Could you check a few things on this model? Use its own coordinates, in mm. Face numbers are marked on the shaded views. Round coordinates to 2 decimals unless told otherwise and drop trailing zeros. Loops run counter-clockwise (first coordinate to the right, second up) from the corner with the lowest first, then second, coordinate; pieces in that order, holes last. Notation, with made-up numbers: (59, 57) - (111, 57) arc R17 ccw to (111, 72) - close; hole circle Ø4 at (22.5, -25.5). An arc over 180 degrees is marked (long way). Answer as CSV lines item,"result". Start each with the question number.
1) Suppose I cut it at C-C, the plane y = -4. Write out the boundary of the cut face in (x, z), then the cut area to 3 significant figures.
2) Please list where these lines run through material, in increasing order: line 1 along X through (y, z) = (-3.65, 0); line 2 along Z through (x, y) = (59.43, -2.5); line 3 along X through (y, z) = (0.5, -5).
3) We'd pull the mould along Z, two halves only. Please class the marked faces 1, 2 and 3: pulls with the +Z half, pulls with the -Z half, needs draft (parallel to the pull), parting line crosses it, or undercut.
4) Suppose I cut it at A-A, the plane x = 59.43. Write out the boundary of the cut face in (y, z).
5) Suppose I cut it at B-B, the plane z = 0. Write out the boundary of the cut face in (x, y).
6) Suppose I cut it at D-D, the plane x = 0. Write out the boundary of the cut face in (y, z).
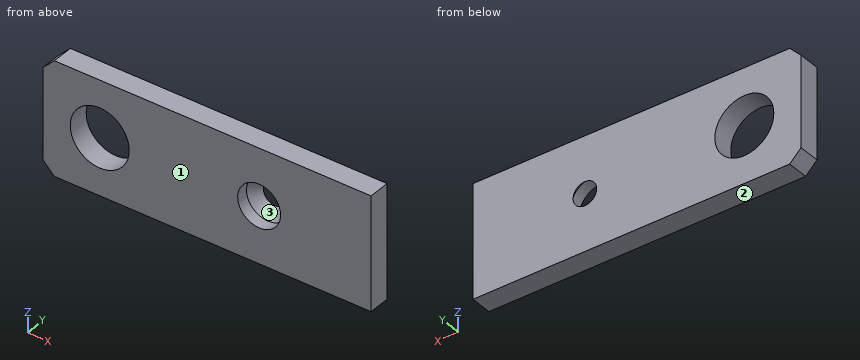
```python
from build123d import *

# Parameters (mm, degrees)
SKETCH1_W           = 42.3
SKETCH1_H           = 42.3
SKETCH1_R           = 11
BOSS_EXTRUDE1_DEPTH = 2
SKETCH2_W           = 80
SKETCH2_H           = 42.3
SKETCH2_R           = 8
BOSS_EXTRUDE2_DEPTH = 2
SKETCH3_W           = 122.3
SKETCH3_H           = 42.3
SKETCH3_R           = 8
SKETCH3_R_2         = 11
BOSS_EXTRUDE3_DEPTH = 6
CUT_EXTRUDE1_DEPTH  = 8


with BuildPart() as part:
    # Sketch1 → Boss-Extrude1 (new body)
    with BuildSketch(Plane(origin=(0, 0, 0), x_dir=(1, 0, 0), z_dir=(0, 1, 0))):
        Rectangle(SKETCH1_W, SKETCH1_H)
        with Locations(Location((0, 0, 0), (0, 0, 270))):
            Circle(SKETCH1_R, mode=Mode.SUBTRACT)
    extrude(amount=BOSS_EXTRUDE1_DEPTH)

    # Sketch2 → Boss-Extrude2 (add)
    with BuildSketch(Plane(origin=(0, 2, 0), x_dir=(1, 0, 0), z_dir=(0, 1, 0))):
        with Locations((61.15, 0)):
            Rectangle(SKETCH2_W, SKETCH2_H)
        with Locations(Location((59.43, 0, 0), (0, 0, 270))):
            Circle(SKETCH2_R, mode=Mode.SUBTRACT)
    extrude(amount=-BOSS_EXTRUDE2_DEPTH)

    # Sketch3 → Boss-Extrude3 (add)
    with BuildSketch(Plane.XZ):
        with Locations((40, 0)):
            Rectangle(SKETCH3_W, SKETCH3_H)
        with Locations(Location((59.43, 0, 0), (0, 0, 90))):
            Circle(SKETCH3_R, mode=Mode.SUBTRACT)
        with Locations(Location((0, 0, 0), (0, 0, 270))):
            Circle(SKETCH3_R_2, mode=Mode.SUBTRACT)
    extrude(amount=BOSS_EXTRUDE3_DEPTH)

    # Sketch5 → Revolve1 (revolve)
    with BuildSketch(Plane.XY, mode=Mode.PRIVATE) as revolve1_sk:
        Polygon((67.43, 2), (63.83, 2), (67.43, -1.6), align=None)
    revolve(revolve1_sk.sketch.rotate(Axis((59.43, 0, 0), (0, 1, 0)), 90), axis=Axis((59.43, 0, 0), (0, 1, 0)))

    # Sketch6 → Cut-Extrude1 (cut)
    with BuildSketch(Plane(origin=(0, 2, 0), x_dir=(1, 0, 0), z_dir=(0, 1, 0))):
        Polygon((-21.15, 16.907359313), (-16.907359313, 21.15), (-21.15, 21.15), align=None)
        Polygon((-21.15, -21.15), (-21.15, -16.907359313), (-16.907359313, -21.15), align=None)
    extrude(amount=-CUT_EXTRUDE1_DEPTH, mode=Mode.SUBTRACT)


solid = part.part
```
Filled sheet:
1,outline,"(-21.15, -16.91) - (-16.91, -21.15) - (101.15, -21.15) - (101.15, 21.15) - (-16.91, 21.15) - (-21.15, 16.91) - close; hole circle Ø22 at (0, 0); hole circle Ø16 at (59.43, 0)"
1,area,"4,570 mm²"
2,line 1,"-21.15 to -11, 11 to 51.43, 67.43 to 101.15"
2,line 2,"-21.15 to -8, 8 to 21.15"
2,line 3,"-21.15 to -9.8, 9.8 to 56.3, 62.56 to 101.15"
3,face 1,"needs draft"
3,face 2,"pulls with the -Z half"
3,face 3,"undercut"
4,outline,"(-6, -21.15) - (2, -21.15) - (2, -4.4) - (-1.6, -8) - (-6, -8) - close; (-6, 8) - (-1.6, 8) - (2, 4.4) - (2, 21.15) - (-6, 21.15) - close"
5,outline,"(-21.15, -6) - (-11, -6) - (-11, 2) - (-21.15, 2) - close; (11, -6) - (51.43, -6) - (51.43, -1.6) - (55.03, 2) - (11, 2) - close; (63.83, 2) - (67.43, -1.6) - (67.43, -6) - (101.15, -6) - (101.15, 2) - close"
6,outline,"(-6, -21.15) - (2, -21.15) - (2, -11) - (-6, -11) - close; (-6, 11) - (2, 11) - (2, 21.15) - (-6, 21.15) - close"
